from build123d import *

# Parameters (mm, degrees)
SKETCH2_W           = 114.3
SKETCH2_H           = 100
SKETCH2_R           = 1.475
SKETCH2_R_2         = 36.5
SKETCH2_W_2         = 19.05
SKETCH2_H_2         = 25.4
BOSS_EXTRUDE1_DEPTH = 0.508
FILLET1_R           = 6.35


with BuildPart() as part:
    # Sketch2 → Boss-Extrude1 (new body)
    # profile 1 of 5: a face of its own
    with BuildSketch(Plane.XY):
        Rectangle(SKETCH2_W, SKETCH2_H)
        with Locations((50.8, 0)):
            Circle(SKETCH2_R, mode=Mode.SUBTRACT)
        with Locations((-50.8, 0)):
            Circle(SKETCH2_R, mode=Mode.SUBTRACT)
        Circle(SKETCH2_R_2, mode=Mode.SUBTRACT)
    # profile 2 of 5: a face of its own
    with BuildSketch(Plane.XY):
        with Locations((-66.675, 16.666666667)):
            Rectangle(SKETCH2_W_2, SKETCH2_H_2)
    # profile 3 of 5: a face of its own
    with BuildSketch(Plane.XY):
        with Locations((-66.675, -16.666666667)):
            Rectangle(SKETCH2_W_2, SKETCH2_H_2)
    # profile 4 of 5: a face of its own
    with BuildSketch(Plane.XY):
        with Locations((66.675, 16.666666667)):
            Rectangle(SKETCH2_W_2, SKETCH2_H_2)
    # profile 5 of 5: a face of its own
    with BuildSketch(Plane.XY):
        with Locations((66.675, -16.666666667)):
            Rectangle(SKETCH2_W_2, SKETCH2_H_2)
    extrude(amount=BOSS_EXTRUDE1_DEPTH)

    # Fillet1
    fillet1_edges = [part.edges().sort_by_distance(p)[0] for p in [
        (76.2, 29.366666667, 0.254),
        (76.2, 3.966666667, 0.254),
        (76.2, -3.966666667, 0.254),
        (76.2, -29.366666667, 0.254),
        (57.15, -50, 0.254),
        (-57.15, -50, 0.254),
        (-76.2, -29.366666667, 0.254),
        (-76.2, -3.966666667, 0.254),
        (-76.2, 3.966666667, 0.254),
        (-76.2, 29.366666667, 0.254),
        (-57.15, 50, 0.254),
        (57.15, 50, 0.254),
    ]]
    fillet(fillet1_edges, radius=FILLET1_R)


solid = part.part
Part model, mm, in its own coordinate system. A direction names the side the tool comes from. Give positions to 0.01 mm unless a question says otherwise; leave off trailing zeros. Loops run counter-clockwise (first coordinate to the right, second up) from the corner with the lowest first, then second, coordinate; pieces in that order, holes last.
(1) Pin check, flat tip, straight feed: pin 1 (1.8 mm diameter, centred on x = 50.8, y = 0, fed in from +Z). Stop position of the tip, or through.
Return value:
pin 1: passes through
(2) Band-saw the part on A-A (x = 0). Write the cut outline in (y, z).
Return value:
outline: (-50, 0) - (-36.5, 0) - (-36.5, 0.51) - (-50, 0.51) - close; (36.5, 0) - (50, 0) - (50, 0.51) - (36.5, 0.51) - close
(3) Band-saw the part on B-B (y = -13.5). Write the cut outline in (x, z).
Return value:
outline: (-76.2, 0) - (-33.91, 0) - (-33.91, 0.51) - (-76.2, 0.51) - close; (33.91, 0) - (76.2, 0) - (76.2, 0.51) - (33.91, 0.51) - close
(4) 3-axis set-ups, long thin cutter, end or side, ignore diameter. For faces 1 (the cylindrical face through (74.29, 5.777, 0.258)), 2 (the cylindrical face through (-55.34, 48.09, 0.26)), 3 (the cylindrical face through (-74.29, 5.777, 0.258)): which of +Z, -Z, +X, -X, +Y, -Y reach the whole face in a straight line?
Return value:
face 1: +Z, -Z, +X
face 2: +Z, -Z, -X, +Y
face 3: +Z, -Z, -X
(5) Drill centre lines: line 1 along Y through (x, z) = (50.8, 0.25) (3 decimals); line 2 along Y through (x, z) = (50.5, 0.1); line 3 along X through (y, z) = (43, 0.1). Where is each one in solid material? Low to high.
Return value:
line 1: y = -50 to -1.475, 1.475 to 50
line 2: y = -50 to -1.44, 1.44 to 50
line 3: x = -57.15 to 57.15
(6) Pull direction X, two halves, no side cores. Call faces 4 (the cylindrical face through (-52.274, 0.065, 0.25)), 5 (the cylindrical face through (55.24, -48.19, 0.26)), 6 (the flat face through (-35, 12, 0)): pulls with the +X half, pulls with the -X half, needs draft (parallel to the pull), parting line crosses it, or undercut.
Return value:
face 4: undercut
face 5: pulls with the +X half
face 6: needs draft
(7) Band-saw the part on C-C (z = 0.3). Count the separate pieces of the cut face and the enclosed holes in it, and give its area (3 significant figures).
Return value:
separate pieces: 1
enclosed holes: 3
area: 9,060 mm2
